Part model, mm, in its own coordinate system. A direction names the side the tool comes from. Give positions to 0.01 mm unless a question says otherwise; leave off trailing zeros. Write each loop counter-clockwise with the first axis right and the second up, starting at its lowest first coordinate (ties: lowest second). Pieces come first, ordered by that corner, then holes.
from build123d import *

# Parameters (mm, degrees)
F1_DEPTH = 6.35


with BuildPart() as f1:
    # F0 (on Front) → F1 (new body)
    with BuildSketch(Plane.XZ):
        with BuildLine():
            Line((0, 19.05), (0, 0))
            Line((0, 0), (6.35, 0))
            ThreePointArc((6.35, 0), (10.840128, 1.859872), (12.7, 6.35))
            Line((12.7, 6.35), (12.7, 30.48))
            ThreePointArc((12.7, 30.48), (10.840128, 34.970128), (6.35, 36.83))
            Line((6.35, 36.83), (-120.65, 36.83))
            ThreePointArc((-120.65, 36.83), (-125.140128, 34.970128), (-127, 30.48))
            Line((-127, 30.48), (-127, 24.13))
            Line((-127, 24.13), (-139.7, 24.13))
            Line((-139.7, 24.13), (-139.7, 36.83))
            ThreePointArc((-139.7, 36.83), (-144.190128, 34.970128), (-146.05, 30.48))
            Line((-146.05, 30.48), (-146.05, 25.4))
            ThreePointArc((-146.05, 25.4), (-144.190128, 20.909872), (-139.7, 19.05))
            Line((-139.7, 19.05), (-114.3, 19.05))
            Line((-114.3, 19.05), (-114.3, 6.35))
            ThreePointArc((-114.3, 6.35), (-112.440128, 1.859872), (-107.95, 0))
            Line((-107.95, 0), (-101.6, 0))
            Line((-101.6, 0), (-101.6, 19.05))
            Line((-101.6, 19.05), (0, 19.05))
        make_face()
    extrude(amount=F1_DEPTH)


solid = f1.part
1) Saw through at C-C (z = 11). Write the cut outline in (x, y).
Check result:
outline: (-114.3, -6.35) - (-101.6, -6.35) - (-101.6, 0) - (-114.3, 0) - close; (0, -6.35) - (12.7, -6.35) - (12.7, 0) - (0, 0) - close
2) Saw through at A-A (z = 29). Write the cut outline in (x, y), and give its area (3 significant figures).
Check result:
outline: (-146.05, -6.35) - (-139.7, -6.35) - (-139.7, 0) - (-146.05, 0) - close; (-127, -6.35) - (12.7, -6.35) - (12.7, 0) - (-127, 0) - close
area: 927 mm2
3) Drill centre lines: L1, parallel to X at y = -5.75, z = 11.5; L2, parallel to X at y = -0.25, z = 29; L3, parallel to Z at x = -92, y = -4.5. Where is each one in solid material? Low to high.
Check result:
L1: x = -114.3 to -101.6, 0 to 12.7
L2: x = -146.05 to -139.7, -127 to 12.7
L3: z = 19.05 to 36.83
4) Saw through at B-B (y = -2). Write the cut outline in (x, z).
Check result:
outline: (-146.05, 25.4) arc R6.35 ccw to (-139.7, 19.05) - (-114.3, 19.05) - (-114.3, 6.35) arc R6.35 ccw to (-107.95, 0) - (-101.6, 0) - (-101.6, 19.05) - (0, 19.05) - (0, 0) - (6.35, 0) arc R6.35 ccw to (12.7, 6.35) - (12.7, 30.48) arc R6.35 ccw to (6.35, 36.83) - (-120.65, 36.83) arc R6.35 ccw to (-127, 30.48) - (-127, 24.13) - (-139.7, 24.13) - (-139.7, 36.83) arc R6.35 ccw to (-146.05, 30.48) - close
5) Saw through at D-D (x = -10.5). Write the cut outline in (y, z).
Check result:
outline: (-6.35, 19.05) - (0, 19.05) - (0, 36.83) - (-6.35, 36.83) - close
6) 3-axis set-ups, long thin cutter, end or side, ignore diameter. For faces 1 (the flat face through (-114.3, -3, 13)), 2 (the flat face through (-133, -3, 24.13)), 3 (the flat face through (-52, -3, 19.05)): which of +Z, -Z, +X, -X, +Y, -Y reach the whole face in a straight line?
Check result:
face 1: -Z, -X, +Y, -Y
face 2: +Z, +Y, -Y
face 3: -Z, +Y, -Y
7) Flat gauge pins, fed straight in: P1, Ø1.9, axis at y = -3, z = 6, coming from the -X side; P2, Ø2, axis at x = -119.5, y = -2, coming from the -Z side. Where does each tip first touch, or does it go through?
Check result:
P1: stops at x = -114.3
P2: stops at z = 19.05
8) Mould opens along X. For faces 4 (the flat face through (-139.7, -3, 30)), 5 (the flat face through (3, -3, 0)), 6 (the cylindrical face through (-112.49, -3.13, 1.91)) say: +X half, -X half, draft (parallel to the pull), parting line (faces both ways), or undercut.
Check result:
face 4: undercut
face 5: draft
face 6: -X half
